```python
from build123d import *

# Parameters (mm, degrees)
BOSS_EXTRUDE1_DEPTH = 1.524


with BuildPart() as part:
    # Sketch1 → Boss-Extrude1 (new body)
    with BuildSketch(Plane.XY):
        with BuildLine():
            Line((0.085387869, 8.76561387), (0.085387869, -0.853085355))
            Line((0.085387869, -0.853085355), (-7.118587452, -0.853085355))
            Line((-7.118587452, -0.853085355), (-9.316419949, 10.53014054))
            Line((-9.316419949, 10.53014054), (-10.812784042, 10.241227919))
            Line((-10.812784042, 10.241227919), (-11.963375606, 16.20048264))
            Line((-11.963375606, 16.20048264), (-10.467011514, 16.489395261))
            Line((-10.467011514, 16.489395261), (-11.318780173, 20.900957592))
            Line((-11.318780173, 20.900957592), (-11.491926915, 21.797735888))
            ThreePointArc((-11.491926915, 21.797735888), (0.847387869, 22.653117291), (13.186702652, 21.797735888))
            Line((13.186702652, 21.797735888), (13.01355591, 20.900957592))
            Line((13.01355591, 20.900957592), (12.161787251, 16.489395261))
            Line((12.161787251, 16.489395261), (13.658151343, 16.20048264))
            Line((13.658151343, 16.20048264), (12.507559779, 10.241227919))
            Line((12.507559779, 10.241227919), (11.011195687, 10.53014054))
            Line((11.011195687, 10.53014054), (8.813363189, -0.853085355))
            Line((8.813363189, -0.853085355), (1.609387869, -0.853085355))
            Line((1.609387869, -0.853085355), (1.609387869, 8.76561387))
            Line((1.609387869, 8.76561387), (0.085387869, 8.76561387))
        make_face()
    extrude(amount=BOSS_EXTRUDE1_DEPTH)


solid = part.part
```
CAD build for the part. Positions are in the model's coordinates, mm. A direction names the side the tool comes from. Round coordinates to 2 decimals unless told otherwise and drop trailing zeros. Loops run counter-clockwise (first coordinate to the right, second up) from the corner with the lowest first, then second, coordinate; pieces in that order, holes last. Notation, with made-up numbers: (-8.5, -24) - (50.5, -24) arc R21 ccw to (50.5, -15) - close; hole circle Ø10 at (-1, 22.5). An arc over 180 degrees is marked (long way). Return JSON: item names as keys, results as strings. Group by question number.
Q1. Tool access for faces 5 (the face through (12.899, 16.347, 0.751)), 6 (the face through (13.1, 13.3, 0.8)), 7 (the face through (0.085, 4, 1)): list every direction of +Z, -Z, +X, -X, +Y, -Y with a clear straight run to the whole face (end or side of a thin tool).
Q2. Flat gauge pin, fed straight in: pin 1 Ø0.5 at (y, z) = (2, 1) entering from -X. Where does the tip first touch, or does it go through?
Q3. Two-plate mould, pull along X, no slides. Class faces 1 (the face through (1.609, 4, 1)), 2 (the face through (1, 14, 0)), 3 (the face through (-11.226, 16.343, 0.751)), 4 (the face through (0.674, 22.653, 0.751)): +X half, -X half, draft (parallel to the pull), parting line (faces both ways), or undercut.
Q4. Band-saw the part on C-C on y = 14.25. Give the cut face in (x, z), plus the area to 3 significant figures.
Q5. Band-saw the part on B-B on x = 10.5. Give the cut face in (y, z).
Q6. Drill centre lines: line 1 along Y through (x, z) = (0, 0.55); line 2 along X through (y, z) = (2, 0.5); line 3 along X through (y, z) = (7.5, 1.25). Where is each one in solid material? Low to high. Write a range as [from, to].
Q7. Band-saw the part on A-A on z = 0.8. Give the cut face in (x, y).
Solutions:
{
 "1": {"face 5": "+Z, -Z, +X", "face 6": "+Z, -Z, +X, -Y", "face 7": "+Z, -Z, -Y"},
 "2": {"pin 1": "stops at x = -7.72"},
 "3": {"face 1": "undercut", "face 2": "draft", "face 3": "-X half", "face 4": "parting line"},
 "4": {"outline": "(-11.59, 0) - (13.28, 0) - (13.28, 1.52) - (-11.59, 1.52) - close", "area": "37.9 mm^2"},
 "5": {"outline": "(7.88, 0) - (22.13, 0) - (22.13, 1.52) - (7.88, 1.52) - close"},
 "6": {"line 1": "y = [-0.85, 22.65]", "line 2": "x = [-7.67, 0.09], [1.61, 9.36]", "line 3": "x = [-8.73, 0.09], [1.61, 10.43]"},
 "7": {"outline": "(-11.96, 16.2) - (-10.81, 10.24) - (-9.32, 10.53) - (-7.12, -0.85) - (0.09, -0.85) - (0.09, 8.77) - (1.61, 8.77) - (1.61, -0.85) - (8.81, -0.85) - (11.01, 10.53) - (12.51, 10.24) - (13.66, 16.2) - (12.16, 16.49) - (13.19, 21.8) arc R89.43 ccw to (-11.49, 21.8) - (-10.47, 16.49) - close"}
}
